from build123d import *

# Parameters (mm, degrees)
Y_KSEKLIK_EKSTR_ZYON1_DEPTH = 1.8923
Y_KSEKLIK_EKSTR_ZYON2_DEPTH = 6.096
KES_EKSTR_ZYON1_DEPTH       = 12.192
KES_EKSTR_ZYON2_DEPTH       = 12.192


with BuildPart() as part:
    # Sketch1 → Y_kseklik-Ekstr_zyon1 (new, symmetric)
    with BuildSketch(Plane(origin=(0, 0, 0), x_dir=(0, 0, -1), z_dir=(1, 0, 0))):
        with BuildLine():
            ThreePointArc((12.43174189, 51.653146377), (10.57551869, 28.624343729), (13.97, 5.771579944))
            Line((13.97, 5.771579944), (12.7, 4.501579944))
            ThreePointArc((12.7, 4.501579944), (6.566277721, 23.771006964), (8.944783318, 43.852741893))
            ThreePointArc((8.944783318, 43.852741893), (10.513707619, 47.830974191), (12.43174189, 51.653146377))
        make_face()
        with BuildLine():
            Line((4.117213446, 13.716), (8.632497279, 13.716))
            ThreePointArc((8.632497279, 13.716), (6.444536578, 25.308553187), (7.160995779, 37.084))
            Line((7.160995779, 37.084), (2.774818776, 37.084))
            ThreePointArc((2.774818776, 37.084), (2.117821696, 25.32370074), (4.117213446, 13.716))
        make_face()
    extrude(amount=Y_KSEKLIK_EKSTR_ZYON1_DEPTH, both=True)

    # Sketch1_3 → Y_kseklik-Ekstr_zyon2 (add, symmetric)
    with BuildSketch(Plane(origin=(0, 0, 0), x_dir=(0, 0, -1), z_dir=(1, 0, 0))):
        with BuildLine():
            ThreePointArc((12.43174189, 51.653146377), (10.57551869, 28.624343729), (13.97, 5.771579944))
            Line((13.97, 5.771579944), (12.7, 4.501579944))
            ThreePointArc((12.7, 4.501579944), (6.566277721, 23.771006964), (8.944783318, 43.852741893))
            ThreePointArc((8.944783318, 43.852741893), (10.513707619, 47.830974191), (12.43174189, 51.653146377))
        make_face()
    extrude(amount=Y_KSEKLIK_EKSTR_ZYON2_DEPTH, both=True)

    # izim1 → Kes-Ekstr_zyon1 (cut)
    with BuildSketch(Plane(origin=(6.096, 0, 0), x_dir=(0, 0, -1), z_dir=(1, 0, 0))):
        Polygon((7.62, 44.45), (15.24, 40.050590949), (15.24, 52.750590949), (7.62, 52.750590949), align=None)
    extrude(amount=-KES_EKSTR_ZYON1_DEPTH, mode=Mode.SUBTRACT)

    # izim2 → Kes-Ekstr_zyon2 (cut)
    with BuildSketch(Plane(origin=(6.096, 0, 0), x_dir=(0, 0, -1), z_dir=(1, 0, 0))):
        Polygon((11.056013618, 42.466216613), (10.070471058, 41.153776474), (10.833720947, 40.007340668), (9.666309047, 38.326799056), (10.636905522, 36.868919313), (9.625699381, 35.413242873), (10.559264156, 34.764728954), (9.31975158, 32.980395197), (10.523316237, 32.05751251), (9.135536699, 30.247659073), (10.564730984, 29.151765592), (9.21036613, 27.202096845), (10.693333077, 26.171932969), (9.442971206, 24.371981166), (10.894662465, 23.363543386), (9.778604553, 21.756928135), (11.145926492, 20.807098693), (10.065994729, 19.252488648), (11.457703408, 18.285718614), (10.75224072, 16.573828628), (11.771303497, 16.153877128), (11.08269787, 14.482892825), (12.125579376, 14.053125727), (11.389100528, 12.265971303), (12.55932158, 11.783728112), (11.974340159, 10.3642004), (12.945895778, 9.963826401), (12.459272873, 8.782977446), (13.296950377, 8.437774058), (12.784445432, 7.194119223), (13.696666966, 6.818196552), (13.362164192, 6.006485377), (13.97, 5.771579944), (16.64122078, 5.771579944), (16.64122078, 42.466216613), align=None)
    extrude(amount=-KES_EKSTR_ZYON2_DEPTH, mode=Mode.SUBTRACT)


solid = part.part
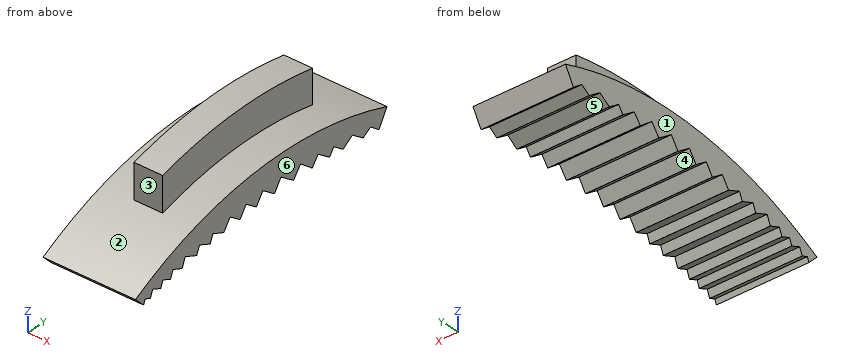
Input: part model. Units: mm. Frame: model coordinates. Face numbers are marked on the shaded views. A direction names the side the tool comes from. Give positions to 0.01 mm unless a question says otherwise; leave off trailing zeros. Loops run counter-clockwise (first coordinate to the right, second up) from the corner with the lowest first, then second, coordinate; pieces in that order, holes last. Notation, with made-up numbers: (-26.75, 47) -> (-10.75, 47) arc R23 cw to (-10.75, 60) -> close; hole circle Ø1 at (3, 47.25). An arc over 180 degrees is marked (long way). Answer as a JSON object with one key per item and string values. Group by question number.
Item 1: Cut plane B-B, the plane y = 39. Return the cut outline in (x, z), and give its area (3 significant figures).
Item 2: Cut plane A-A, the plane z = -8.25. Return the cut outline in (x, y), and give its area (3 significant figures).
Item 3: Pull-direction query (Y, two-part tool) for the marked faces 1, 2, 3 and 4; classes: released by +Y, released by -Y, zero draft, split by the parting line, or undercut.
Item 4: Cut plane C-C, the plane z = -5.75. Return the cut outline in (x, y).
Item 5: Reachability of the marked faces 5 and 6 from +Z, -Z, +X, -X, +Y, -Y: full face, straight path, thin tool, end or side. Return the list, or none.
Item 6: Pin query (flat end, axial travel): P1, Ø2, axis at x = 1, y = 27, coming from the +Z side; P2, Ø4, axis at x = -0.5, z = -4, coming from the +Y side. Return the tip coordinate at first contact, or that it passes through.
Item 7: Line query: probe 1 along Y at (x, z) = (-1.5, -11.5); probe 2 along Y at (x, z) = (0, -6.75); probe 3 along X at (y, z) = (35, -6). Output: solid intervals per line, ascending.
Checks:
{
 "1": {"outline": "(-6.1, -10.13) -> (6.1, -10.13) -> (6.1, -7.56) -> (-6.1, -7.56) -> close", "area": "31.4 mm²"},
 "2": {"outline": "(-6.1, 14.97) -> (-1.89, 14.97) -> (-1.89, 13.72) -> (1.89, 13.72) -> (1.89, 14.97) -> (6.1, 14.97) -> (6.1, 41.66) -> (-6.1, 41.66) -> close", "area": "330 mm²"},
 "3": {"face 1": "zero draft", "face 2": "split by the parting line", "face 3": "released by -Y", "face 4": "undercut"},
 "4": {"outline": "(-1.89, 13.72) -> (1.89, 13.72) -> (1.89, 37.08) -> (-1.89, 37.08) -> close"},
 "5": {"face 5": "-Z, +X, -X", "face 6": "+Z, -Z, +X, +Y, -Y"},
 "6": {"P1": "stops at z = -2.03", "P2": "stops at y = 37.08"},
 "7": {"probe 1": "y = 6.73 to 12.22, 12.54 to 14.31, 15.5 to 16.27", "probe 2": "y = 13.72 to 37.08", "probe 3": "x = -1.89 to 1.89"}
}
